Geometry check sheet. Reference: the model listing, model coordinates, mm. Round coordinates to 2 decimals unless told otherwise and drop trailing zeros. Order: outer loops, then holes, each group sorted by start corner. A loop starts at its lowest first (then second) coordinate and runs counter-clockwise, first axis right, second up.
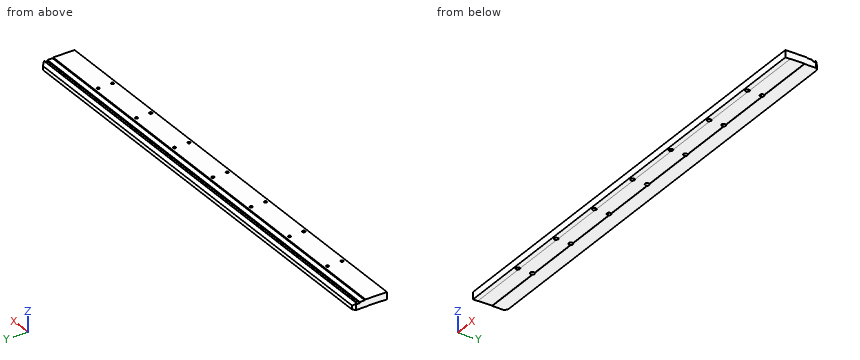
```python
from build123d import *

# Parameters (mm, degrees)
F0_W           = 14.224
F0_H           = 20.574
F1_DEPTH       = 1244.6
F3_D           = 14.2875
F3_CBORE_D     = 21.43125
F3_CBORE_DEPTH = 13.49375
F4_SIZE        = 12.7


# Not quite as in the source:
# - a length typed as a fraction of an inch, garbled in the dataset ("3 / 203.2 mm" for 3/8 in), is restored


with BuildPart() as f1:
    # F0 (on Right) → F1 (new body, symmetric)
    with BuildSketch(Plane.YZ):
        Polygon((26.162, 19.05), (-88.138, 19.05), (-88.138, -19.05), (-62.738, -19.05), (-62.738, -17.526), (13.462, -17.526), (13.462, -19.05), (73.914, -19.05), (73.914, 1.524), (88.138, 1.524), (73.66, 16.002), (72.136, 16.002), (72.136, 9.652), (56.388, 9.652), (56.388, 16.002), (29.21, 16.002), align=None)
        with Locations((81.026, -8.763)):
            Rectangle(F0_W, F0_H)
    extrude(amount=F1_DEPTH, both=True)

    # F3 (through all)
    with Locations(Plane(origin=(0, 0, -19.05), x_dir=(1, 0, 0), z_dir=(0, 0, -1))):
        with Locations((914.4, -7.112), (914.4, 69.088), (609.6, 69.088), (609.6, -7.112), (304.8, -7.112), (304.8, 69.088), (0, -7.112), (0, 69.088), (-304.8, -7.112), (-304.8, 69.088), (-609.6, -7.112), (-609.6, 69.088), (-914.4, -7.112), (-914.4, 69.088)):
            CounterBoreHole(F3_D / 2, F3_CBORE_D / 2, F3_CBORE_DEPTH)

    # F4
    f4_edges = [f1.edges().sort_by_distance(p)[0] for p in [
        (1244.6, 88.138, -8.763),
        (-1244.6, 88.138, -8.763),
    ]]
    chamfer(f4_edges, length=F4_SIZE)


solid = f1.part
```
(1) Depth check by flat-ended pin: P1, Ø17, axis at x = -914.4, y = -69.088, coming from the -Z side; P2, Ø1.7, axis at x = 366.5, y = 73, coming from the +Z side; P3, Ø1, axis at x = -954.5, y = -47.5, coming from the -Z side. Enter the tip coordinate at first touch or a pass-through.
Returned:
P1: stops at z = -5.56
P2: stops at z = 16
P3: stops at z = -17.53
(2) Material ranges on line 1 (Y direction, x = 914, z = -8); line 2 (Y direction, x = 0, z = 10.25); line 3 (Z direction, x = -1045.5, y = 54.5), recorded low to high.
Returned:
line 1: y = -88.14 to -79.8, -58.38 to -3.6, 17.82 to 88.14
line 2: y = -88.14 to -76.23, -61.94 to -0.03, 14.26 to 56.39, 72.14 to 79.41
line 3: z = -19.05 to 16
(3) Sectioned sample at A-A, the plane x = -561. Record the cut outline in (y, z), and give its area (3 significant figures).
Returned:
outline: (-88.14, -19.05) - (-62.74, -19.05) - (-62.74, -17.53) - (13.46, -17.53) - (13.46, -19.05) - (88.14, -19.05) - (88.14, 1.52) - (73.66, 16) - (72.14, 16) - (72.14, 9.65) - (56.39, 9.65) - (56.39, 16) - (29.21, 16) - (26.16, 19.05) - (-88.14, 19.05) - close
area: 6,210 mm2
